Check sheet for the drawn part. Datum: minimum x, y, z corner. Units: mm. A direction names the side the tool comes from. Give positions to 0.01 mm unless a question says otherwise; leave off trailing zeros. Write each loop counter-clockwise with the first axis right and the second up, starting at its lowest first coordinate (ties: lowest second). Pieces come first, ordered by that corner, then holes. Notation, with made-up numbers: (4, 1) -> (50, 1) arc R6 ccw to (50, 7) -> close; hole circle Ø4 at (36.5, 54). An arc over 180 degrees is marked (long way). Answer as CSV lines item,"result". Start each with the question number.
1) Material ranges on L1, parallel to Y at x = 27, z = 74.5 (3 decimals); L2, parallel to Z at x = 37, y = 34.5 (3 decimals); L3, parallel to Z at x = 109, y = 19.5 (3 decimals), recorded low to high.
2) Sectioned sample at C-C on x = 42.5. Record the cut outline in (y, z) (3 decimals), and give its area (3 significant figures).
3) Sectioned sample at B-B on z = 55. Record the cut outline in (x, y) (1 decimal).
4) Sectioned sample at A-A on y = 13.5. Record the cut outline in (x, z) (1 decimal).
5) Sectioned sample at D-D on z = 21. Record the cut outline in (x, y) (1 decimal), and give its area (3 significant figures).
6) Gauge pin test, flat ends, axial feed: pin 1 Ø1.5 at (x, y) = (113, 33) entering from +Z (3 decimals); pin 2 Ø17 at (x, z) = (44, 25.5) entering from -Y; pin 3 Ø9.5 at (x, y) = (34, 25) entering from -Z. Record the tip position at first contact, or that the pin passes through.
7) Tool access check on the marked faces 4, 5 and 6. Record the directions out of +Z, -Z, +X, -X, +Y, -Y that give a thin tool (end or side, any length) a straight path to the whole face; none if there is none.
8) Mould release check, pull along X, two halves, no side actions. Record for the marked faces 1, 2 and 3: released by +X, released by -X, zero draft, split by the parting line, or undercut.
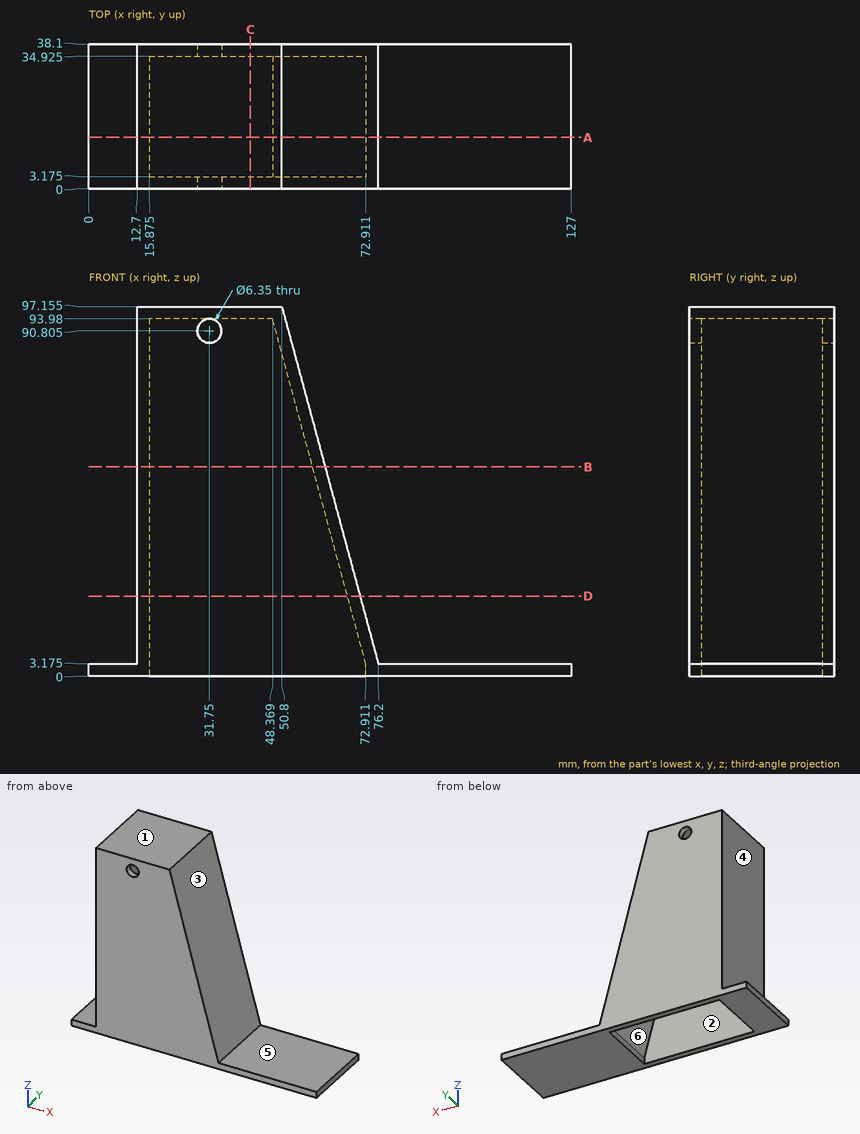
Ans:
1,L1,"y = 0 to 3.175, 34.925 to 38.1"
1,L2,"z = 93.98 to 97.155"
1,L3,"z = 0 to 3.175"
2,outline,"(0, 0) -> (3.175, 0) -> (3.175, 93.98) -> (34.925, 93.98) -> (34.925, 0) -> (38.1, 0) -> (38.1, 97.155) -> (0, 97.155) -> close"
2,area,"718 mm²"
3,outline,"(12.7, 0) -> (62.2, 0) -> (62.2, 38.1) -> (12.7, 38.1) -> close; hole (15.9, 3.2) -> (58.9, 3.2) -> (58.9, 34.9) -> (15.9, 34.9) -> close"
4,outline,"(0, 0) -> (15.9, 0) -> (15.9, 94) -> (48.4, 94) -> (72.9, 3.2) -> (72.9, 0) -> (127, 0) -> (127, 3.2) -> (76.2, 3.2) -> (50.8, 97.2) -> (12.7, 97.2) -> (12.7, 3.2) -> (0, 3.2) -> close"
5,outline,"(12.7, 0) -> (71.4, 0) -> (71.4, 38.1) -> (12.7, 38.1) -> close; hole (15.9, 3.2) -> (68.1, 3.2) -> (68.1, 34.9) -> (15.9, 34.9) -> close"
5,area,"578 mm²"
6,pin 1,"stops at z = 3.175"
6,pin 2,"stops at y = 0"
6,pin 3,"stops at z = 93.98"
7,face 4,"+Z, -X, +Y, -Y"
7,face 5,"+Z, +X, +Y, -Y"
7,face 6,"-Z"
8,face 1,"zero draft"
8,face 2,"undercut"
8,face 3,"released by +X"
